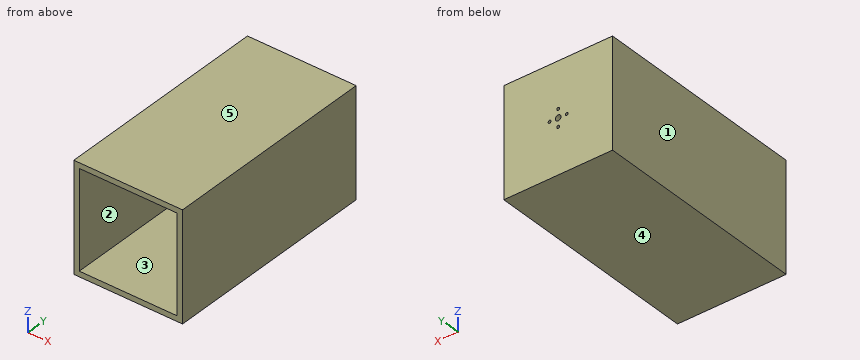
from build123d import *

# Parameters (mm, degrees)
SKETCH1_W           = 76.2
SKETCH1_H           = 152.4
BOSS_EXTRUDE1_DEPTH = 76.2
SKETCH2_W           = 68.58
SKETCH2_H           = 68.58
CUT_EXTRUDE1_DEPTH  = 148.59
SKETCH3_R           = 2
SKETCH3_R_2         = 1
CUT_EXTRUDE2_DEPTH  = 153.4


with BuildPart() as part:
    # Sketch1 → Boss-Extrude1 (new body)
    with BuildSketch(Plane.XY):
        with Locations((38.1, 76.2)):
            Rectangle(SKETCH1_W, SKETCH1_H)
    extrude(amount=-BOSS_EXTRUDE1_DEPTH)

    # Sketch2 → Cut-Extrude1 (cut)
    with BuildSketch(Plane.XZ):
        with Locations((38.1, -38.1)):
            Rectangle(SKETCH2_W, SKETCH2_H)
    extrude(amount=-CUT_EXTRUDE1_DEPTH, mode=Mode.SUBTRACT)

    # Sketch3 → Cut-Extrude2 (cut, through all)
    with BuildSketch(Plane(origin=(0, 152.4, 0), x_dir=(1, 0, 0), z_dir=(0, 1, 0))):
        with Locations((38.1, 38.1)):
            Circle(SKETCH3_R)
        with Locations((38.1, 44.1)):
            Circle(SKETCH3_R_2)
        with Locations((38.1, 32.1)):
            Circle(SKETCH3_R_2)
        with Locations((44.1, 38.1)):
            Circle(SKETCH3_R_2)
        with Locations((32.1, 38.1)):
            Circle(SKETCH3_R_2)
    extrude(amount=-CUT_EXTRUDE2_DEPTH, mode=Mode.SUBTRACT)


solid = part.part
Here's how the part is built. I have some questions about the finished solid (model axes, mm). Face numbers are marked on the shaded views. A direction names the side the tool comes from. Coordinates: 2 decimals unless noted, no trailing zeros. Order: outer loops, then holes, each group sorted by start corner. A loop starts at its lowest first (then second) coordinate and runs counter-clockwise, first axis right, second up. Notation, with made-up numbers: M 36.25,31 L 89.25,31 A10 ccw 89.25,47 Z; hole C 23,83 d7. An arc over 180 degrees is marked long. Answer as CSV lines item,"result".
Item 1: For pin 1 (6.5 mm diameter, centred on x = 38.1, z = -38.1, fed in from -Y); pin 2 (4 mm diameter, centred on y = 74.5, z = -60, fed in from -X), each with a flat end and sliding along its axis, tell me the tip position at first contact or that it passes through.
Results found:
pin 1,"y = 148.59"
pin 2,"x = 0"
Item 2: Imagine slicing it at B-B on z = -59.5. Write out the boundary of the cut face in (x, y), plus the area to 3 significant figures.
Results found:
outline,"M 0,0 L 3.81,0 L 3.81,148.59 L 72.39,148.59 L 72.39,0 L 76.2,0 L 76.2,152.4 L 0,152.4 Z"
area,"1,420 mm2"
Item 3: If I drill on line 1 (X direction, y = 151, z = -38); line 2 (Z direction, x = 32.1, y = 149.65); line 3 (Z direction, x = 38.1, y = 150.45), over which ranges is the centre line in solid material (lowest first)?
Results found:
line 1,"0 to 31.11, 33.09 to 36.1, 40.1 to 43.11, 45.09 to 76.2"
line 2,"-76.2 to -39.1, -37.1 to 0"
line 3,"-76.2 to -45.1, -43.1 to -40.1, -36.1 to -33.1, -31.1 to 0"
Item 4: On a 3-axis mill with a long thin cutter (end or side, diameter ignored), from which of +Z, -Z, +X, -X, +Y, -Y can I reach the whole of each face in a straight line? I mean the marked faces 1 and 2. Say none if no direction works.
Results found:
face 1,"+Z, -Z, -X, +Y, -Y"
face 2,"-Y"
Item 5: Imagine slicing it at C-C on x = 15.5. Write out the boundary of the cut face in (y, z), plus the area to 3 significant figures.
Results found:
outline,"M 0,-76.2 L 152.4,-76.2 L 152.4,0 L 0,0 L 0,-3.81 L 148.59,-3.81 L 148.59,-72.39 L 0,-72.39 Z"
area,"1,420 mm2"
Item 6: Imagine slicing it at A-A on y = 129. Write out the boundary of the cut face in (x, z), plus the area to 3 significant figures.
Results found:
outline,"M 0,-76.2 L 76.2,-76.2 L 76.2,0 L 0,0 Z; hole M 3.81,-72.39 L 72.39,-72.39 L 72.39,-3.81 L 3.81,-3.81 Z"
area,"1,100 mm2"
Item 7: We'd pull the mould along Z, two halves only. Please class the marked faces 3, 4 and 5: +Z half, -Z half, draft (parallel to the pull), parting line (faces both ways), or undercut.
Results found:
face 3,"undercut"
face 4,"-Z half"
face 5,"+Z half"
